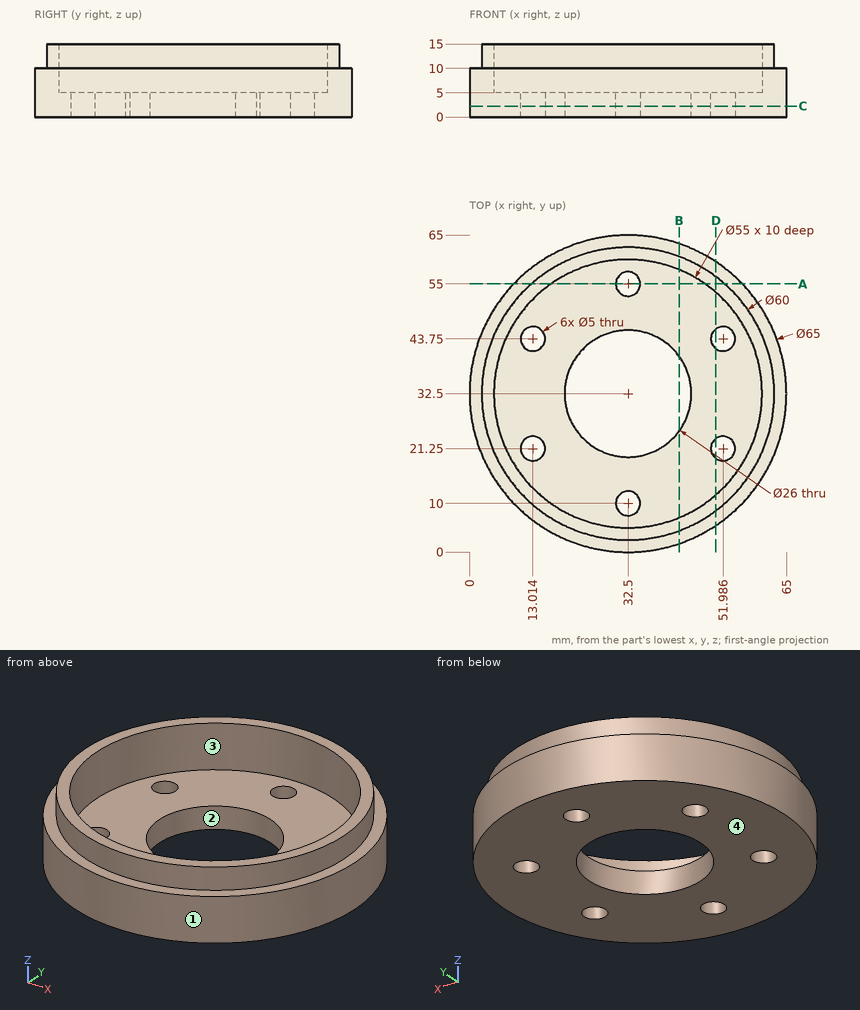
Drawing for the job (mm, zero at the part's lowest x, y, z). Give positions to 0.01 mm unless a question says otherwise; leave off trailing zeros. Loops run counter-clockwise (first coordinate to the right, second up) from the corner with the lowest first, then second, coordinate; pieces in that order, holes last.
(1) Band-saw the part on B-B (x = 43). Write the cut outline in (y, z) (1 decimal).
Return value:
outline: (1.7, 0) - (24.8, 0) - (24.8, 5) - (7.1, 5) - (7.1, 15) - (4.4, 15) - (4.4, 10) - (1.7, 10) - close; (40.2, 0) - (63.3, 0) - (63.3, 10) - (60.6, 10) - (60.6, 15) - (57.9, 15) - (57.9, 5) - (40.2, 5) - close
(2) Drill centre lines: line 1 along Y through (x, z) = (32.5, 1.95); line 2 along Y through (x, z) = (52, 2.75); line 3 along Y through (x, z) = (34.5, 1) (1 decimal). Where is each one in solid material? Low to high.
Return value:
line 1: y = 0 to 7.5, 12.5 to 19.5, 45.5 to 52.5, 57.5 to 65
line 2: y = 6.5 to 18.75, 23.75 to 41.25, 46.25 to 58.5
line 3: y = 0.1 to 8.5, 11.5 to 19.7, 45.3 to 53.5, 56.5 to 64.9
(3) Band-saw the part on D-D (x = 50.5). Write the cut outline in (y, z), and give its area (3 significant figures).
Return value:
outline: (5.44, 0) - (19.24, 0) - (19.24, 5) - (11.71, 5) - (11.71, 15) - (8.5, 15) - (8.5, 10) - (5.44, 10) - close; (23.26, 0) - (41.74, 0) - (41.74, 5) - (23.26, 5) - close; (45.76, 0) - (59.56, 0) - (59.56, 10) - (56.5, 10) - (56.5, 15) - (53.29, 15) - (53.29, 5) - (45.76, 5) - close
area: 325 mm2
(4) Band-saw the part on A-A (y = 55). Write the cut outline in (x, z).
Return value:
outline: (9.05, 0) - (30, 0) - (30, 5) - (16.69, 5) - (16.69, 15) - (12.66, 15) - (12.66, 10) - (9.05, 10) - close; (35, 0) - (55.95, 0) - (55.95, 10) - (52.34, 10) - (52.34, 15) - (48.31, 15) - (48.31, 5) - (35, 5) - close
(5) Band-saw the part on C-C (z = 2.25). Count the separate pieces of the cut face and the enclosed holes in it, and give its area (3 significant figures).
Return value:
separate pieces: 1
enclosed holes: 7
area: 2,670 mm2
(6) Pull direction X, two halves, no side cores. Call the marked faces 1, 2, 3 and 4: pulls with the +X half, pulls with the -X half, needs draft (parallel to the pull), parting line crosses it, or undercut.
Return value:
face 1: parting line crosses it
face 2: undercut
face 3: undercut
face 4: needs draft
(7) Pin check, flat tips, straight feed: pin 1 (4 mm diameter, centred on x = 32.5, y = 10, fed in from -Z); pin 2 (1 mm diameter, centred on x = 52, y = 18, fed in from +Z); pin 3 (6 mm diameter, centred on x = 36.5, z = 2.5, fed in from +Y) (1 decimal); pin 4 (2 mm diameter, centred on x = 10, z = 11.5, fed in from +Y). Stop position of each tip, or through.
Return value:
pin 1: passes through
pin 2: stops at z = 5
pin 3: stops at y = 65
pin 4: stops at y = 53.42
